The drawing under review shows one solid part. Ordinate dimensions are in mm from its lowest x, y, z. A direction names the side the tool comes from. Give positions to 0.01 mm unless a question says otherwise; leave off trailing zeros. Loops run counter-clockwise (first coordinate to the right, second up) from the corner with the lowest first, then second, coordinate; pieces in that order, holes last.
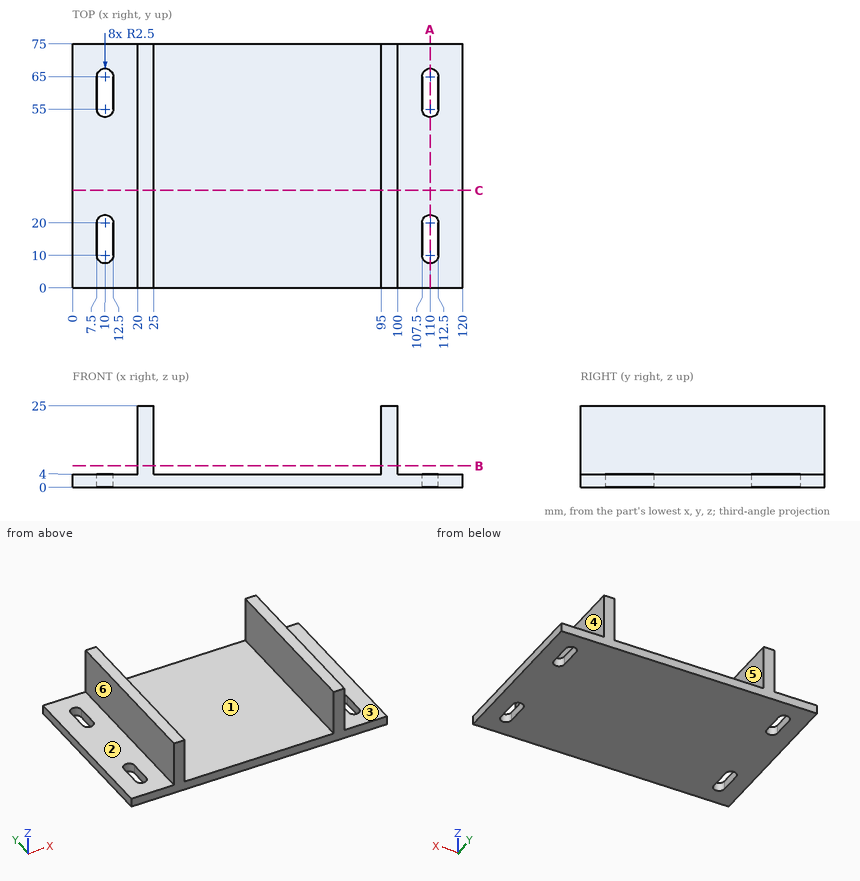
Item 1: For L1, parallel to X at y = 47.5, z = 24; L2, parallel to X at y = 8, z = 2.25; L3, parallel to Z at x = 34, y = 62.5, list the stretches that pass through material, from the lowest coordinate up.
Answer:
L1: x = 20 to 25, 95 to 100
L2: x = 0 to 8.5, 11.5 to 108.5, 111.5 to 120
L3: z = 0 to 4
Item 2: Clearance check with flat-ended pins moving along their axes: pin 1 Ø10 at (y, z) = (47.5, 22) entering from -X; pin 2 Ø8 at (x, z) = (88, 19) entering from -Y; pin 3 Ø12 at (x, y) = (48.5, 54.5) entering from +Z. State where each tip first meets the part, or that it passes through.
Answer:
pin 1: stops at x = 20
pin 2: passes through
pin 3: stops at z = 4
Item 3: Take a section at A-A on x = 110. Give the boundary of the cut face in (y, z).
Answer:
outline: (0, 0) - (7.5, 0) - (7.5, 4) - (0, 4) - close; (22.5, 0) - (52.5, 0) - (52.5, 4) - (22.5, 4) - close; (67.5, 0) - (75, 0) - (75, 4) - (67.5, 4) - close
Item 4: Tool access review of the marked faces 1, 2 and 3: name each direction out of +Z, -Z, +X, -X, +Y, -Y from which nothing blocks a thin tool from reaching the whole face with its end or side.
Answer:
face 1: +Z, +Y, -Y
face 2: +Z, -X, +Y, -Y
face 3: +Z, +X, +Y, -Y
Item 5: Take a section at C-C on y = 30. Give the boundary of the cut face in (x, z), and give its area (3 significant figures).
Answer:
outline: (0, 0) - (120, 0) - (120, 4) - (100, 4) - (100, 25) - (95, 25) - (95, 4) - (25, 4) - (25, 25) - (20, 25) - (20, 4) - (0, 4) - close
area: 690 mm2
Item 6: The part is to be moulded in two halves that separate along X. For the marked faces 4, 5 and 6, say which applies: released by +X, released by -X, zero draft, split by the parting line, or undercut.
Answer:
face 4: released by +X
face 5: undercut
face 6: released by -X
Item 7: Take a section at B-B on z = 6.5. Give the boundary of the cut face in (x, y), and give its area (3 significant figures).
Answer:
outline: (20, 0) - (25, 0) - (25, 75) - (20, 75) - close; (95, 0) - (100, 0) - (100, 75) - (95, 75) - close
area: 750 mm2
